from build123d import *

# Parameters (mm, degrees)
SKETCH_R        = 60
SKETCH_R_2      = 7.5
SKETCH_R_3      = 3.2
SKETCH_R_4      = 5.05
PAD_DEPTH       = 14
SKETCH001_R     = 70
POCKET_DEPTH    = 3.5
POCKET001_DEPTH = 4
SKETCH003_R     = 6.5
POCKET002_DEPTH = 7.5
CHAMFER_SIZE    = 1


with BuildPart() as part:
    # Sketch → Pad (new body)
    with BuildSketch(Plane.XY):
        Circle(SKETCH_R)
        Circle(SKETCH_R_2, mode=Mode.SUBTRACT)
        with Locations((21.92031, 21.92031)):
            Circle(SKETCH_R_3, mode=Mode.SUBTRACT)
        with Locations((-52, 0)):
            Circle(SKETCH_R_4, mode=Mode.SUBTRACT)
        with Locations((52, 0)):
            Circle(SKETCH_R_4, mode=Mode.SUBTRACT)
        with Locations((0, 52)):
            Circle(SKETCH_R_4, mode=Mode.SUBTRACT)
        with Locations((0, -52)):
            Circle(SKETCH_R_4, mode=Mode.SUBTRACT)
    extrude(amount=PAD_DEPTH)

    # Sketch001 → Pocket (cut)
    with BuildSketch(Plane(origin=(0, 0, 0), x_dir=(1, 0, 0), z_dir=(0, 0, -1))):
        Circle(SKETCH001_R)
        with BuildLine():
            ThreePointArc((-41.534414, 15.11729), (-44.2, 0), (-41.534414, -15.11729))
            Line((-41.534414, -15.11729), (-47.924324, -17.443027))
            ThreePointArc((-47.924324, -17.443027), (-36.062446, -36.062446), (-17.443027, -47.924324))
            Line((-15.11729, -41.534414), (-17.443027, -47.924324))
            ThreePointArc((-15.11729, -41.534414), (0, -44.2), (15.11729, -41.534414))
            Line((15.11729, -41.534414), (17.443027, -47.924324))
            ThreePointArc((17.443027, -47.924324), (36.062446, -36.062446), (47.924324, -17.443027))
            Line((41.534414, -15.11729), (47.924324, -17.443027))
            ThreePointArc((41.534414, -15.11729), (44.2, 0), (41.534414, 15.11729))
            Line((41.534414, 15.11729), (47.924324, 17.443027))
            ThreePointArc((47.924324, 17.443027), (36.062446, 36.062446), (17.443027, 47.924324))
            Line((15.11729, 41.534414), (17.443027, 47.924324))
            ThreePointArc((15.11729, 41.534414), (0, 44.2), (-15.11729, 41.534414))
            Line((-15.11729, 41.534414), (-17.443027, 47.924324))
            ThreePointArc((-17.443027, 47.924324), (-36.062446, 36.062446), (-47.924324, 17.443027))
            Line((-41.534414, 15.11729), (-47.924324, 17.443027))
        make_face(mode=Mode.SUBTRACT)
    extrude(amount=-POCKET_DEPTH, mode=Mode.SUBTRACT)

    # Sketch002 → Pocket001 (cut)
    with BuildSketch(Plane.XY.offset(14)):
        with BuildLine():
            Line((4.644542, -15.439722), (81.321028, 65.300484))
            Line((81.321028, 65.300484), (64.32339, 80.393113))
            Line((64.32339, 80.393113), (-15.439722, 4.644542))
            ThreePointArc((-15.439722, 4.644542), (-15.702333, -15.702333), (4.644542, -15.439722))
        make_face()
    extrude(amount=-POCKET001_DEPTH, mode=Mode.SUBTRACT)

    # Sketch003 → Pocket002 (cut)
    with BuildSketch(Plane.XY.offset(14)):
        with Locations((0, 52)):
            Circle(SKETCH003_R)
        with Locations((52, 0)):
            Circle(SKETCH003_R)
        with Locations((0, -52)):
            Circle(SKETCH003_R)
        with Locations((-52, 0)):
            Circle(SKETCH003_R)
    extrude(amount=-POCKET002_DEPTH, mode=Mode.SUBTRACT)

    # Chamfer
    chamfer_edges = [part.edges().sort_by_distance(p)[0] for p in [
        (8.612883, 27.486561, 14),
    ]]
    chamfer(chamfer_edges, length=CHAMFER_SIZE)


solid = part.part
The listing builds one solid part. Answer for the finished solid, in the listing's coordinates (mm). A direction names the side the tool comes from. Give positions to 0.01 mm unless a question says otherwise; leave off trailing zeros. Write each loop counter-clockwise with the first axis right and the second up, starting at its lowest first coordinate (ties: lowest second). Pieces come first, ordered by that corner, then holes. Notation, with made-up numbers: (81.5, -12) -> (129.5, -12) arc R14 ccw to (129.5, 9) -> close; hole circle Ø8 at (30, 50). An arc over 180 degrees is marked (long way). One line per question, with ' | ' between items. Start each with the question number.
1. Section B-B (x = -51) is taken. Determine the outline of the cut face in (y, z).
2. Section A-A (z = 11.5) is taken. Determine the outline of the cut face in (x, y).
3. Section C-C (y = 9) is taken. Determine the outline of the cut face in (x, z), plus the area to 3 significant figures.
4. Find the intervals of material crossed by probe 1 along X at (y, z) = (0, 4.1); probe 2 along Y at (x, z) = (-1.5, 6), in increasing order.
5. Section D-D (x = -30) is taken. Determine the outline of the cut face in (y, z).
6. For a pull along Y with two mould halves and no side action, classify faces 1 (the flat face through (-16.264, 44.685, 1.726)), 2 (the cylindrical face through (-57.045, 0.222, 4.979)), 3 (the cylindrical face through (-59.94, 2.64, 8.68)) as pulls with the +Y half, pulls with the -Y half, needs draft (parallel to the pull), parting line crosses it, or undercut.
7. For faces 4 (the flat face through (8.95, 27.806, 11.521)), 5 (the cylindrical face through (0.2, -44.2, 1.7)), 6 (the cylindrical face through (-0.2, 44.2, 1.7)), 7 (the cylindrical face through (-35.841, -36.282, 1.726)), determine the directions among +Z, -Z, +X, -X, +Y, -Y from which every point of the face is accessible in a straight line to the end or side of a thin tool.
8. Given pin 1 Ø4 at (x, z) = (27.5, 12) entering from -Y; pin 2 Ø6 at (x, y) = (21.92, 21.92) entering from +Z; pin 3 Ø6 at (x, z) = (-1.5, 3.5) entering from -Y; pin 4 Ø1 at (y, z) = (-1.5, 5.5) entering from -X, each flat-ended and moving along its own axis, determine where each tip first touches the part or whether it passes through.
Response values:
1) outline: (-31.61, 3.5) -> (-4.95, 3.5) -> (-4.95, 6.5) -> (-6.42, 6.5) -> (-6.42, 14) -> (-31.61, 14) -> close; (4.95, 3.5) -> (31.61, 3.5) -> (31.61, 14) -> (6.42, 14) -> (6.42, 6.5) -> (4.95, 6.5) -> close
2) outline: (-15.44, 4.64) -> (32.67, 50.33) arc R60 ccw (long way) to (50.33, 32.67) -> (4.64, -15.44) arc R14.21 cw (long way) to start; hole circle Ø13 at (-52, 0); hole circle Ø13 at (0, -52); hole circle Ø13 at (0, 52); hole circle Ø13 at (52, 0)
3) outline: (-59.32, 3.5) -> (-43.27, 3.5) -> (-43.27, 0) -> (43.27, 0) -> (43.27, 3.5) -> (59.32, 3.5) -> (59.32, 14) -> (29.23, 14) -> (27.85, 13) -> (27.85, 10) -> (-10.85, 10) -> (-10.85, 13) -> (-12.31, 14) -> (-59.32, 14) -> close | area: 1,390 mm2
4) probe 1: -60 to -57.05, -46.95 to -7.5, 7.5 to 46.95, 57.05 to 60 | probe 2: -59.98 to -56.82, -47.18 to -7.35, 7.35 to 47.18, 56.82 to 59.98
5) outline: (-51.96, 3.5) -> (-41.24, 3.5) -> (-41.24, 0) -> (41.24, 0) -> (41.24, 3.5) -> (51.96, 3.5) -> (51.96, 14) -> (-51.96, 14) -> close
6) face 1: pulls with the +Y half | face 2: undercut | face 3: parting line crosses it
7) face 4: +Z | face 5: -Z, -Y | face 6: -Z, +Y | face 7: -Z, -X, -Y
8) pin 1: y = -54.31 | pin 2: through | pin 3: y = -60 | pin 4: x = -59.99
